from build123d import *

# Parameters (mm, degrees)
SKETCH_1_W          = 15
SKETCH_1_H          = 3
SKETCH_1_W_2        = 3
SKETCH_1_H_2        = 15
EXTRUDE_1_DEPTH     = 3
SKETCH_2_R          = 2
CUT_EXTRUDE_1_DEPTH = 3


with BuildPart() as part:
    # 草图1 → 凸台-拉伸1 (new body)
    with BuildSketch(Plane(origin=(0, 0, 0), x_dir=(1, 0, 0), z_dir=(0, 1, 0))):
        Polygon((28, -21.5), (28, -1.5), (7.5, -1.5), (-7.5, -1.5), (-22.5, -1.5), align=None)
        Rectangle(SKETCH_1_W, SKETCH_1_H)
        with Locations((21.5, 21)):
            Rectangle(SKETCH_1_W_2, SKETCH_1_H_2)
        with Locations((21.5, 56)):
            Rectangle(SKETCH_1_W_2, SKETCH_1_H_2)
        Polygon((46.671361037, -21.5), (28, -21.5), (28, -1.5), (28, 1.5), (23, 1.5), (23, 13.5), (23, 28.5), (23, 48.5), (23, 63.5), (23, 73.5), (81.889727457, 39.5), align=None)
        Polygon((-22.5, -1.5), (-22.5, -9.5), (28, -21.5), align=None)
    extrude(amount=EXTRUDE_1_DEPTH)

    # 草图2 → 切除-拉伸1 (cut)
    with BuildSketch(Plane(origin=(0, 3, 0), x_dir=(1, 0, 0), z_dir=(0, 1, 0))):
        with Locations(Location((63.229473419, 27.179491924, 0), (0, 0, 270))):
            Circle(SKETCH_2_R)
        with Locations(Location((55.729473419, 14.189110868, 0), (0, 0, 270))):
            Circle(SKETCH_2_R)
        with Locations(Location((48.229473419, 1.198729811, 0), (0, 0, 270))):
            Circle(SKETCH_2_R)
    extrude(amount=-CUT_EXTRUDE_1_DEPTH, mode=Mode.SUBTRACT)


solid = part.part
CAD build for the part. Positions are in the model's coordinates, mm. A direction names the side the tool comes from. Round coordinates to 2 decimals unless told otherwise and drop trailing zeros. Loops run counter-clockwise (first coordinate to the right, second up) from the corner with the lowest first, then second, coordinate; pieces in that order, holes last. Notation, with made-up numbers: (28.5, 75.5) - (48.5, 75.5) arc R27 cw to (48.5, 91.5) - close; hole circle Ø2 at (38, 78.5). An arc over 180 degrees is marked (long way). Put each result on its own line as item: value.
1. Slice it at B-B on z = -46.5. List the corners of the cut face in (x, y).
Geometry check:
outline: (23, 0) - (69.77, 0) - (69.77, 3) - (23, 3) - close
2. Slice it at A-A on y = 0.5. List the corners of the cut face in (x, z), and give its area (3 significant figures).
Geometry check:
outline: (-22.5, 1.5) - (-7.5, 1.5) - (-7.5, -1.5) - (7.5, -1.5) - (7.5, 1.5) - (28, 1.5) - (28, -1.5) - (23, -1.5) - (23, -13.5) - (20, -13.5) - (20, -28.5) - (23, -28.5) - (23, -48.5) - (20, -48.5) - (20, -63.5) - (23, -63.5) - (23, -73.5) - (81.89, -39.5) - (46.67, 21.5) - (28, 21.5) - (-22.5, 9.5) - close; hole circle Ø4 at (48.23, -1.2); hole circle Ø4 at (55.73, -14.19); hole circle Ø4 at (63.23, -27.18)
area: 4,210 mm²
3. 3-axis set-ups, long thin cutter, end or side, ignore diameter. For faces 4 (the flat face through (21, 1, -28.5)), 5 (the flat face through (23, 1, -68)), 6 (the flat face through (26, 1, -1.5)): which of +Z, -Z, +X, -X, +Y, -Y reach the whole face in a straight line?
Geometry check:
face 4: -X, +Y, -Y
face 5: -Z, -X, +Y, -Y
face 6: +Y, -Y
4. Wall check: line 1 (X direction, y = 0.8, z = -1); line 2 (Z direction, x = 47.5, y = 0.5); line 3 (Z direction, x = 49, y = 1.15). Give the ranges that are in metal, low to high.
Geometry check:
line 1: -7.5 to 7.5, 28 to 46.24, 50.22 to 59.66
line 2: -59.35 to -3.06, 0.66 to 20.06
line 3: -58.49 to -3.04, 0.65 to 17.47
5. Two-plate mould, pull along Z, no slides. Class faces 1 (the flat face through (37, 1, 21.5)), 2 (the flat face through (23, 1, -38)), 3 (the flat face through (7.5, 1, 0)): released by +Z, released by -Z, zero draft, split by the parting line, or undercut.
Geometry check:
face 1: released by +Z
face 2: undercut
face 3: zero draft
6. Pin check, flat tips, straight feed: P1, Ø1.5, axis at x = 25.5, y = 1.5, coming from the +Z side; P2, Ø0.9, axis at x = 22, y = 1, coming from the -Z side; P3, Ø0.9, axis at y = 2, z = 0, coming from the -X side. Stop position of each tip, or through.
Geometry check:
P1: z = 21.08
P2: z = -63.5
P3: x = -7.5
7. Slice it at C-C on x = 36.5. List the corners of the cut face in (y, z), and give its area (3 significant figures).
Geometry check:
outline: (0, -65.71) - (3, -65.71) - (3, 21.5) - (0, 21.5) - close
area: 262 mm²
